The model under review builds one solid part; all positions refer to its coordinate system, in mm. Face numbers are marked on the shaded views. Coordinates: 2 decimals unless noted, no trailing zeros. Write each loop counter-clockwise with the first axis right and the second up, starting at its lowest first coordinate (ties: lowest second). Pieces come first, ordered by that corner, then holes. Notation, with made-up numbers: (30.25, 9) -> (85.25, 9) arc R5 ccw to (85.25, 13) -> close; hole circle Ø11 at (64, 34.5). An arc over 180 degrees is marked (long way). Write each question's results on one line, items separated by ' | '.
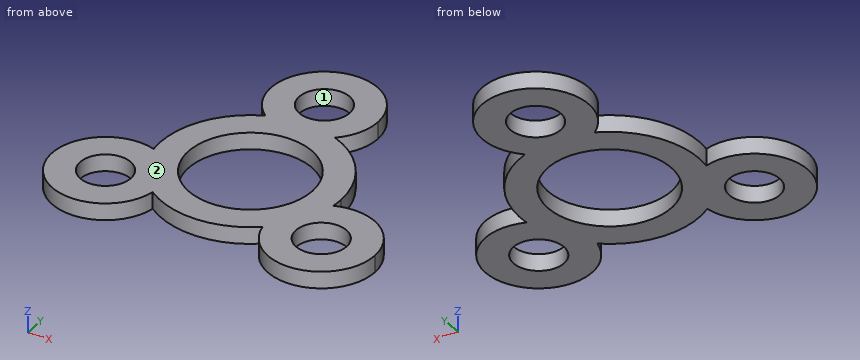
```python
from build123d import *

# Parameters (mm, degrees)
F0_R     = 4.500000108
F0_R_2   = 11
F1_DEPTH = 3


with BuildPart() as f1:
    # F0 (on Top) → F1 (new body)
    with BuildSketch(Plane.XY):
        with BuildLine():
            ThreePointArc((6.1590883621, 14.7670455174), (8.624422863, 18.0163672007), (9.5, 22))
            ThreePointArc((9.5, 22), (-3.9836327993, 30.624422863), (-6.1590883621, 14.7670455174))
            ThreePointArc((-6.1590883621, 14.7670455174), (0, 16.0000000864), (6.1590883621, 14.7670455174))
        make_face()
        with Locations((0, 22)):
            Circle(F0_R, mode=Mode.SUBTRACT)
        with BuildLine():
            ThreePointArc((6.1590883621, 14.7670455174), (0, 16.0000000864), (-6.1590883621, 14.7670455174))
            ThreePointArc((-6.1590883621, 14.7670455174), (0, 12.5), (6.1590883621, 14.7670455174))
        make_face()
        with BuildLine():
            ThreePointArc((6.1590883621, 14.7670455174), (0, 12.5), (-6.1590883621, 14.7670455174))
            ThreePointArc((-6.1590883621, 14.7670455174), (-13.8564065354, 8.0000000432), (-15.868180738, -2.0495957729))
            ThreePointArc((-15.868180738, -2.0495957729), (-11.2904202482, -5.5228471073), (-9.5525588833, -11))
            ThreePointArc((-9.5525588833, -11), (-9.5917731912, -11.8622842279), (-9.7090923758, -12.7174497444))
            ThreePointArc((-9.7090923758, -12.7174497444), (0, -16.0000000864), (9.7090923758, -12.7174497444))
            ThreePointArc((9.7090923758, -12.7174497444), (10.8253175473, -6.25), (15.868180738, -2.0495957729))
            ThreePointArc((15.868180738, -2.0495957729), (15.967011241, -1.0269151831), (16.0000000864, 0))
            ThreePointArc((16.0000000864, 0), (13.3143797657, 8.8728402566), (6.1590883621, 14.7670455174))
        make_face()
        Circle(F0_R_2, mode=Mode.SUBTRACT)
        with BuildLine():
            ThreePointArc((-9.7090923758, -12.7174497444), (-13.8564065354, -8.0000000432), (-15.868180738, -2.0495957729))
            ThreePointArc((-15.868180738, -2.0495957729), (-27.2798002192, -15.75), (-9.7090923758, -12.7174497444))
        make_face()
        with Locations((-19.0525588833, -11)):
            Circle(F0_R, mode=Mode.SUBTRACT)
        with BuildLine():
            ThreePointArc((-9.5525588833, -11), (-11.2904202482, -5.5228471073), (-15.868180738, -2.0495957729))
            ThreePointArc((-15.868180738, -2.0495957729), (-13.8564065354, -8.0000000432), (-9.7090923758, -12.7174497444))
            ThreePointArc((-9.7090923758, -12.7174497444), (-9.5917731912, -11.8622842279), (-9.5525588833, -11))
        make_face()
        with BuildLine():
            ThreePointArc((9.7090923758, -12.7174497444), (13.8564065354, -8.0000000432), (15.868180738, -2.0495957729))
            ThreePointArc((15.868180738, -2.0495957729), (10.8253175473, -6.25), (9.7090923758, -12.7174497444))
        make_face()
        with BuildLine():
            ThreePointArc((28.5525588833, -11), (24.5297117759, -3.2378613649), (15.868180738, -2.0495957729))
            ThreePointArc((15.868180738, -2.0495957729), (13.8564065354, -8.0000000432), (9.7090923758, -12.7174497444))
            ThreePointArc((9.7090923758, -12.7174497444), (19.9148431112, -20.460785692), (28.5525588833, -11))
        make_face()
        with Locations((19.0525588833, -11)):
            Circle(F0_R, mode=Mode.SUBTRACT)
    extrude(amount=F1_DEPTH)


with BuildPart() as f2_1:
    # F2: copy of F1
    add(f1.part.moved(Location((0, 0, 10))))


solid = f1.part
```
Q1. Draft analysis for pull direction X (two halves, no side actions). For the marked faces 1 and 2, state which applies: pulls with the +X half, pulls with the -X half, needs draft (parallel to the pull), parting line crosses it, or undercut.
Solution:
face 1: undercut | face 2: needs draft
Q2. Clearance check with flat-ended pins moving along their axes: P1, Ø1.5, axis at x = -13, z = 2.5, coming from the +Y side; P2, Ø8, axis at x = 19.05, y = -11, coming from the +Z side. State where each tip first meets the part, or that it passes through.
Solution:
P1: y = 10.29 | P2: through
Q3. For line 1 (X direction, y = -14, z = 2); line 2 (X direction, y = -14.5, z = 1.9); line 3 (Y direction, x = -5, z = 2.15), list the stretches that pass through material, from the lowest coordinate up. Write a range as from..to.
Solution:
line 1: -28.07..-22.41, -15.7..-10.04, -7.75..7.75, 10.04..15.7, 22.41..28.07 | line 2: -27.88..-21.88, -16.22..-10.22, -6.76..6.76, 10.22..16.22, 21.88..27.88 | line 3: -15.2..-9.8, 9.8..30.08
Q4. Add section B-B (z = 1.4). Write out the cut boundary in (x, y).
Solution:
outline: (-15.87, -2.05) arc R9.5 ccw (long way) to (-9.71, -12.72) arc R16 ccw to (9.71, -12.72) arc R9.5 ccw (long way) to (15.87, -2.05) arc R16 ccw to (6.16, 14.77) arc R9.5 ccw (long way) to (-6.16, 14.77) arc R16 ccw to start; hole circle Ø9 at (-19.05, -11); hole circle Ø22 at (0, 0); hole circle Ø9 at (0, 22); hole circle Ø9 at (19.05, -11)
Q5. Add section A-A (y = 7). Write out the cut boundary in (x, z), plus the area to 3 significant figures.
Solution:
outline: (-14.39, 0) -> (-8.49, 0) -> (-8.49, 3) -> (-14.39, 3) -> close; (8.49, 0) -> (14.39, 0) -> (14.39, 3) -> (8.49, 3) -> close | area: 35.4 mm²
Q6. Add section C-C (x = -21.5). Write out the cut boundary in (y, z).
Solution:
outline: (-20.18, 0) -> (-14.78, 0) -> (-14.78, 3) -> (-20.18, 3) -> close; (-7.22, 0) -> (-1.82, 0) -> (-1.82, 3) -> (-7.22, 3) -> close
